Can you work these out from the model? Positions are in its coordinate system, mm. A direction names the side the tool comes from. Give positions to 0.01 mm unless a question says otherwise; leave off trailing zeros. Order: outer loops, then holes, each group sorted by start corner. A loop starts at its lowest first (then second) coordinate and runs counter-clockwise, first axis right, second up. Notation, with made-up numbers: (37, 50.5) - (68, 50.5) arc R36 cw to (68, 87.5) - close; hole circle Ø3 at (39.5, -36.5). An arc over 180 degrees is marked (long way). Answer as CSV lines item,"result".
```python
from build123d import *

# Parameters (mm, degrees)
SKETCH1_W                = 180
SKETCH1_H                = 180
BOSS_EXTRUDE1_DEPTH      = 6
SKETCH2_R                = 50.3
SKETCH2_R_2              = 46.3
BOSS_EXTRUDE2_DEPTH      = 19
CUT_EXTRUDE1_DEPTH       = 256.266527379
CUT_EXTRUDE1_DEPTH_BACK  = 256.266527379
SKETCH3_R                = 47
BOSS_EXTRUDE3_DEPTH      = 60
FILLET4_R                = 3
M5_CLEARANCE_HOLE1_D     = 5.5
SKETCH15_W               = 25
SKETCH15_H               = 7
BOSS_EXTRUDE5_DEPTH      = 19
CUT_EXTRUDE3_DEPTH       = 2
FILLET5_R                = 1.5
CUT_EXTRUDE4_REACH       = 264.975
CUT_EXTRUDE5_REACH       = 244.499
SKETCH33_W               = 1
SKETCH33_H               = 25
SKETCH35_W               = 15
SKETCH35_H               = 13
BOSS_EXTRUDE6_DEPTH      = 13
M5_CLEARANCE_HOLE2_D     = 5.5
CUT_EXTRUDE6_DEPTH       = 4.2
CUT_EXTRUDE7_REACH       = 242.936
SKETCH41_W               = 23
SKETCH41_H               = 15
FILLET8_R                = 1
CUT_EXTRUDE8_REACH       = 197.694
SKETCH47_R               = 53
CUT_EXTRUDE10_DEPTH      = 1.12
CUT_EXTRUDE12_DEPTH      = 238.295626108
CUT_EXTRUDE12_DEPTH_BACK = 238.295626108
SKETCH51_W               = 150
SKETCH51_H               = 200
SKETCH52_W               = 25
SKETCH52_H               = 7
SKETCH52_W_2             = 23
SKETCH52_H_2             = 5
BOSS_EXTRUDE9_DEPTH      = 3
CHAMFER1_SIZE            = 1


with BuildPart() as part:
    # Sketch1 → Boss-Extrude1 (new body)
    with BuildSketch(Plane.XY):
        with Locations((90, 90)):
            Rectangle(SKETCH1_W, SKETCH1_H)
    extrude(amount=BOSS_EXTRUDE1_DEPTH)

    # Sketch2 → Boss-Extrude2 (add)
    with BuildSketch(Plane(origin=(0, 0, 0), x_dir=(-1, 0, 0), z_dir=(0, 0, -1))):
        with Locations((-90, 90)):
            Circle(SKETCH2_R)
        with Locations((-90, 90)):
            Circle(SKETCH2_R_2, mode=Mode.SUBTRACT)
    extrude(amount=BOSS_EXTRUDE2_DEPTH)

    # Sketch3 → Cut-Extrude1 (cut, two sides: drawn at the far end of the back side and taken through both)
    with BuildSketch(Plane(origin=(0, 0, 0), x_dir=(-1, 0, 0), z_dir=(0, 0, -1)).offset(-CUT_EXTRUDE1_DEPTH_BACK)):
        with Locations((-90, 90)):
            Circle(SKETCH3_R)
    extrude(amount=CUT_EXTRUDE1_DEPTH + CUT_EXTRUDE1_DEPTH_BACK, mode=Mode.SUBTRACT)

    # Sketch4 → Boss-Extrude3 (add)
    with BuildSketch(Plane(origin=(0, 0, 0), x_dir=(-1, 0, 0), z_dir=(0, 0, -1))):
        with BuildLine():
            Line((0, 77.5), (0, 102.5))
            Line((0, 102.5), (-41.277931078, 102.5))
            ThreePointArc((-41.277931078, 102.5), (-39.7, 90), (-41.277931078, 77.5))
            Line((-41.277931078, 77.5), (0, 77.5))
        make_face()
    extrude(amount=BOSS_EXTRUDE3_DEPTH)

    # Fillet4
    fillet4_edges = [part.edges().sort_by_distance(p)[0] for p in [
        (41.277931078, 102.5, -9.5),
        (41.277931078, 77.5, -9.5),
    ]]
    fillet(fillet4_edges, radius=FILLET4_R)

    # M5 Clearance Hole1 (through all)
    with Locations(Plane(origin=(0, 0, 0), x_dir=(-1, 0, 0), z_dir=(0, 0, -1))):
        with Locations((-107.470285544, 155.199993275), (-155.199993275, 107.470285544), (-155.199993275, 72.529714456), (-107.470285544, 24.800006725), (-72.529714456, 24.800006725), (-24.800006725, 72.529714456), (-24.800006725, 107.470285544), (-72.529714456, 155.199993275)):
            Hole(M5_CLEARANCE_HOLE1_D / 2)

    # Sketch15 → Boss-Extrude5 (add)
    with BuildSketch(Plane(origin=(0, 0, 0), x_dir=(-1, 0, 0), z_dir=(0, 0, -1))):
        with Locations((-149.8, 90)):
            Rectangle(SKETCH15_W, SKETCH15_H)
    extrude(amount=BOSS_EXTRUDE5_DEPTH)

    # Sketch17 → Cut-Extrude3 (cut, symmetric)
    with BuildSketch(Plane(origin=(0, 90, 0), x_dir=(0, 0, -1), z_dir=(0, 1, 0))):
        Polygon((19, -154.732971354), (-1.044131231, -134.688840123), (-5.544131231, -134.688840123), (19, -159.232971354), align=None)
        Polygon((-5.544131231, -134.688840123), (-1.044131231, -134.688840123), (19, -154.732971354), (19, -159.232971354), align=None)
    extrude(amount=CUT_EXTRUDE3_DEPTH, both=True, mode=Mode.SUBTRACT)

    # Fillet5
    fillet5_edges = [part.edges().sort_by_distance(p)[0] for p in [
        (145.845199441, 92, -10.112228087),
        (145.845199441, 88, -10.112228087),
        (148.095199441, 92, -7.862228087),
        (148.095199441, 88, -7.862228087),
    ]]
    fillet(fillet5_edges, radius=FILLET5_R)

    # Sketch31 → Cut-Extrude4 (cut, up to next)
    with BuildSketch(Plane.XY.offset(6), mode=Mode.PRIVATE) as cut_extrude4_sk1:
        with BuildLine():
            Line((0, 180), (0, 102.5))
            Line((0, 102.5), (16.049002711, 102.5))
            ThreePointArc((16.049002711, 102.5), (165, 90), (16.049002711, 77.5))
            Line((16.049002711, 77.5), (0, 77.5))
            Line((0, 77.5), (0, 0))
            Line((0, 0), (180, 0))
            Line((180, 0), (180, 180))
            Line((180, 180), (0, 180))
        make_face()
    cut_extrude4_tool1 = extrude(cut_extrude4_sk1.sketch, amount=-CUT_EXTRUDE4_REACH, mode=Mode.PRIVATE) & part.part
    add(cut_extrude4_tool1.solids().sort_by_distance((2.545584, 141.25, 6))[0], mode=Mode.SUBTRACT)

    # Sketch33 → Cut-Extrude5 (cut, up to next)
    with BuildSketch(Plane.XY.offset(6), mode=Mode.PRIVATE) as cut_extrude5_sk1:
        with Locations((0.5, 90)):
            Rectangle(SKETCH33_W, SKETCH33_H)
    cut_extrude5_tool1 = extrude(cut_extrude5_sk1.sketch, amount=-CUT_EXTRUDE5_REACH, mode=Mode.PRIVATE) & part.part
    add(cut_extrude5_tool1.solids().sort_by_distance((0.5, 90, 6))[0], mode=Mode.SUBTRACT)

    # Sketch35 → Boss-Extrude6 (add)
    with BuildSketch(Plane(origin=(0, 0, 0), x_dir=(-1, 0, 0), z_dir=(0, 0, -1))):
        with Locations((-90, 146.23771205)):
            Rectangle(SKETCH35_W, SKETCH35_H)
        with Locations((-90, 33.76228795)):
            Rectangle(SKETCH35_W, SKETCH35_H)
    extrude(amount=BOSS_EXTRUDE6_DEPTH)

    # M5 Clearance Hole2 (through all)
    with Locations(Plane(origin=(97.5, 0, 0), x_dir=(0, 0, -1), z_dir=(1, 0, 0))):
        with Locations((6.5, 146.23771205), (6.5, 33.76228795)):
            Hole(M5_CLEARANCE_HOLE2_D / 2)

    # Sketch40 → Cut-Extrude6 (cut)
    with BuildSketch(Plane.ZY.offset(-82.5)):
        Polygon((-10.75, 143.783973406), (-6.5, 141.330234762), (-2.25, 143.783973406), (-2.25, 148.691450694), (-6.5, 151.145189338), (-10.75, 148.691450694), align=None)
        Polygon((-2.25, 31.308549306), (-2.25, 36.216026594), (-6.5, 38.669765238), (-10.75, 36.216026594), (-10.75, 31.308549306), (-6.5, 28.854810662), align=None)
    extrude(amount=-CUT_EXTRUDE6_DEPTH, mode=Mode.SUBTRACT)

    # Sketch41 → Cut-Extrude7 (cut, up to next)
    with BuildSketch(Plane(origin=(0, 0, 0), x_dir=(-1, 0, 0), z_dir=(0, 0, -1)), mode=Mode.PRIVATE) as cut_extrude7_sk1:
        with Locations((-90, 160.23771205)):
            Rectangle(SKETCH41_W, SKETCH41_H)
    cut_extrude7_tool1 = extrude(cut_extrude7_sk1.sketch, amount=-CUT_EXTRUDE7_REACH, mode=Mode.PRIVATE) & part.part
    # Sketch41 → Cut-Extrude7 (cut, up to next)
    with BuildSketch(Plane(origin=(0, 0, 0), x_dir=(-1, 0, 0), z_dir=(0, 0, -1)), mode=Mode.PRIVATE) as cut_extrude7_sk2:
        with Locations((-90, 19.76228795)):
            Rectangle(SKETCH41_W, SKETCH41_H)
    cut_extrude7_tool2 = extrude(cut_extrude7_sk2.sketch, amount=-CUT_EXTRUDE7_REACH, mode=Mode.PRIVATE) & part.part
    add(cut_extrude7_tool1.solids().sort_by_distance((90, 160.237712, 0))[0], mode=Mode.SUBTRACT)
    add(cut_extrude7_tool2.solids().sort_by_distance((90, 19.762288, 0))[0], mode=Mode.SUBTRACT)

    # Fillet8
    fillet8_edges = [part.edges().sort_by_distance(p)[0] for p in [
        (101.5, 164.113089262, 3),
        (78.5, 164.113089262, 3),
        (78.5, 15.886910738, 3),
        (101.5, 15.886910738, 3),
    ]]
    fillet(fillet8_edges, radius=FILLET8_R)

    # Sketch42 → Cut-Extrude8 (cut, up to next)
    with BuildSketch(Plane(origin=(0, 102.5, 0), x_dir=(1, 0, 0), z_dir=(0, 1, 0)), mode=Mode.PRIVATE) as cut_extrude8_sk1:
        Polygon((15, -6), (1, 24), (1, -6), align=None)
    cut_extrude8_tool1 = extrude(cut_extrude8_sk1.sketch, amount=-CUT_EXTRUDE8_REACH, mode=Mode.PRIVATE) & part.part
    add(cut_extrude8_tool1.solids().sort_by_distance((5.666667, 102.5, -4))[0], mode=Mode.SUBTRACT)

    # Sketch47 → Cut-Extrude10 (cut)
    with BuildSketch(Plane.XY.offset(6)):
        with Locations((90, 90)):
            Circle(SKETCH47_R)
    extrude(amount=-CUT_EXTRUDE10_DEPTH, mode=Mode.SUBTRACT)

    # Sketch51 → Cut-Extrude12 (cut, two sides: drawn at the far end of the back side and taken through both)
    with BuildSketch(Plane(origin=(0, 0, -13), x_dir=(-1, 0, 0), z_dir=(0, 0, -1)).offset(-CUT_EXTRUDE12_DEPTH_BACK)):
        with Locations((-15, 90)):
            Rectangle(SKETCH51_W, SKETCH51_H)
    extrude(amount=CUT_EXTRUDE12_DEPTH + CUT_EXTRUDE12_DEPTH_BACK, mode=Mode.SUBTRACT)

    # Sketch52 → Boss-Extrude9 (add)
    with BuildSketch(Plane(origin=(0, 0, -19), x_dir=(-1, 0, 0), z_dir=(0, 0, -1))):
        with Locations((-149.8, 90)):
            Rectangle(SKETCH52_W, SKETCH52_H)
        with Locations((-149.8, 90)):
            Rectangle(SKETCH52_W_2, SKETCH52_H_2, mode=Mode.SUBTRACT)
    extrude(amount=BOSS_EXTRUDE9_DEPTH)

    # Chamfer1
    chamfer1_edges = [part.edges().sort_by_distance(p)[0] for p in [
        (161.3, 90, -22),
        (149.8, 87.5, -22),
        (138.3, 90, -22),
        (149.8, 92.5, -22),
    ]]
    chamfer(chamfer1_edges, length=CHAMFER1_SIZE - 0.0001)  # a hair under: the kernel refuses the full size


solid = part.part
```
1) I want a section at B-B on y = 62. Write out the boundary of the cut face in (x, z), plus the area to 3 significant figures.
Answer block:
outline,"(127.75, -19) - (131.79, -19) - (131.79, 0) - (159.58, 0) - (159.58, 6) - (135, 6) - (135, 4.88) - (127.75, 4.88) - close"
area,"260 mm2"
2) I'm going to push flat-ended pins straight in: P1, Ø3, axis at y = 124, z = -10.5, coming from the +X side; P2, Ø14.5, axis at y = 36.5, z = -9, coming from the +X side; P3, Ø4.5, axis at x = 155.2, y = 72.53, coming from the -Z side; P4, Ø4, axis at y = 109.5, z = -3, coming from the -X side. Where does each tip first touch, or does it pass through?
Answer block:
P1,"x = 128.39"
P2,"x = 109.77"
P3,"through"
P4,"x = 131.79"
3) I want a section at C-C on z = -6.5. Count the separate pieces of the cut face and the enclosed holes in it, plus the area to 3 significant figures.
Answer block:
separate pieces,"3"
enclosed holes,"1"
area,"750 mm2"
4) If we mould it in two halves opening along X, with no side actions, what happens to faces 1 (the flat face through (97.5, 146.1, -3.5)), 2 (the cylindrical face through (146.02, 91.57, -9.65)), 3 (the flat face through (94, 34, -13))? For each: +X half, -X half, draft (parallel to the pull), parting line (faces both ways), or undercut.
Answer block:
face 1,"+X half"
face 2,"undercut"
face 3,"draft"
5) I need wall thicknesses on line 1 along Y through (x, z) = (105, 0.25); line 2 along Z through (x, y) = (110.5, 27); line 3 along Z through (x, y) = (138.5, 86). Which ranges of each line are inside material? Lowest first, please. Write a range as [from, to].
Answer block:
line 1,"[16.52, 23.59], [26.01, 45.46], [134.54, 153.99], [156.41, 163.48]"
line 2,"[0, 6]"
line 3,"[-19, 4.88]"
6) I want a section at A-A on x = 118. Write out the boundary of the cut face in (y, z).
Answer block:
outline,"(20.42, 0) - (48.21, 0) - (48.21, -19) - (52.25, -19) - (52.25, 4.88) - (45, 4.88) - (45, 6) - (20.42, 6) - close; (127.75, -19) - (131.79, -19) - (131.79, 0) - (159.58, 0) - (159.58, 6) - (135, 6) - (135, 4.88) - (127.75, 4.88) - close"
7) Which directions (+Z, -Z, +X, -X, +Y, -Y) give clear straight access to the entire face, cutting with the end or side of a thin tool? Please do faces 4 (the flat face through (101.5, 158, 3)), 5 (the flat face through (150, 86.5, -11)), 6 (the cylindrical face through (147.97, 88.45, -8.34)).
Answer block:
face 4,"+Z, -Z, -X, +Y"
face 5,"-Z, +X, -Y"
face 6,"none"
8) I want a section at D-D on x = 129.5. Write out the boundary of the cut face in (y, z).
Answer block:
outline,"(26.24, 0) - (58.86, 0) - (58.86, -19) - (64.53, -19) - (64.53, 4.88) - (54.66, 4.88) - (54.66, 6) - (26.24, 6) - close; (115.47, -19) - (121.14, -19) - (121.14, 0) - (153.76, 0) - (153.76, 6) - (125.34, 6) - (125.34, 4.88) - (115.47, 4.88) - close"
